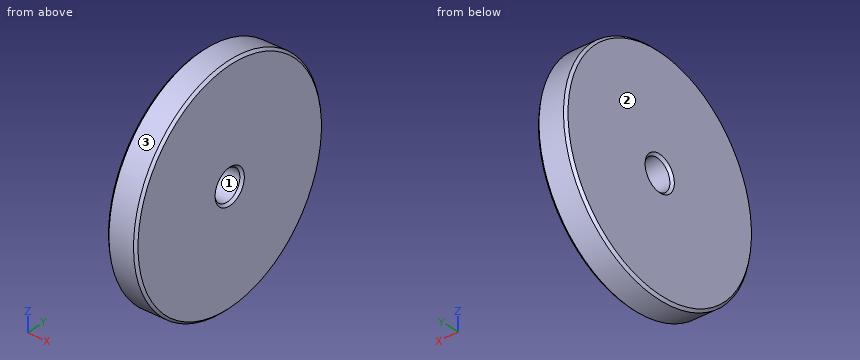
```python
from build123d import *

# Parameters (mm, degrees)
SKETCH1_W        = 12
SKETCH1_H        = 40.25
SFAZOWANIE1_SIZE = 1


with BuildPart() as part:
    # Sketch1 → Base-Revolve (revolve)
    with BuildSketch(Plane.XY, mode=Mode.PRIVATE) as base_revolve_sk:
        with Locations((-7.238439554, 26.375)):
            Rectangle(SKETCH1_W, SKETCH1_H)
    revolve(base_revolve_sk.sketch.rotate(Axis((-17.903027245, 0, 0), (1, 0, 0)), 90), axis=Axis((-17.903027245, 0, 0), (1, 0, 0)))

    # Sfazowanie1
    sfazowanie1_edges = [part.edges().sort_by_distance(p)[0] for p in [
        (-1.238439554, 0, -6.25),
        (-1.238439554, 0, -46.5),
        (-13.238439554, 0, -46.5),
        (-13.238439554, 0, -6.25),
    ]]
    chamfer(sfazowanie1_edges, length=SFAZOWANIE1_SIZE)


solid = part.part
```
Geometry check sheet. Reference: the model listing, model coordinates, mm. Face numbers are marked on the shaded views. Round coordinates to 2 decimals unless told otherwise and drop trailing zeros. Write each loop counter-clockwise with the first axis right and the second up, starting at its lowest first coordinate (ties: lowest second). Pieces come first, ordered by that corner, then holes. Notation, with made-up numbers: (25.25, 15) -> (46.25, 15) arc R16 cw to (46.25, 44) -> close; hole circle Ø6 at (80, -17.75). An arc over 180 degrees is marked (long way). Put each result on its own line as item: value.
1) Thickness scan on probe 1 along Y at (x, z) = (-7.5, 0); probe 2 along Y at (x, z) = (-2.75, 1.5); probe 3 along Z at (x, y) = (-2.75, 41.5). Record the ranges inside material, lowest first. Write a range as from..to.
Recorded:
probe 1: y = -46.5..-6.25, 6.25..46.5
probe 2: y = -46.48..-6.07, 6.07..46.48
probe 3: z = -20.98..20.98
2) Depth check by flat-ended pin: P1, Ø3, axis at x = -11, y = -11, coming from the -Z side; P2, Ø2, axis at x = -2.5, z = 22, coming from the -Y side; P3, Ø1, axis at x = -11, y = -8.5, coming from the +Z side. Enter the tip coordinate at first touch or a pass-through.
Recorded:
P1: stops at z = -45.52
P2: stops at y = -41.49
P3: stops at z = 45.81
3) Cross-section at C-C, the plane x = -10.75. Enter the section's corners in (y, z).
Recorded:
outline: circle Ø93 at (0, 0); hole circle Ø12.5 at (0, 0)
4) Cross-section at A-A, the plane y = 0. Enter the section's corners in (x, z).
Recorded:
outline: (-13.24, -45.5) -> (-12.24, -46.5) -> (-2.24, -46.5) -> (-1.24, -45.5) -> (-1.24, -7.25) -> (-2.24, -6.25) -> (-12.24, -6.25) -> (-13.24, -7.25) -> close; (-13.24, 7.25) -> (-12.24, 6.25) -> (-2.24, 6.25) -> (-1.24, 7.25) -> (-1.24, 45.5) -> (-2.24, 46.5) -> (-12.24, 46.5) -> (-13.24, 45.5) -> close
5) Release check for a two-part mould opening along Z. For the marked faces 1, 2 and 3 record: pulls with the +Z half, pulls with the -Z half, needs draft (parallel to the pull), parting line crosses it, or undercut.
Recorded:
face 1: undercut
face 2: needs draft
face 3: parting line crosses it
